Print and shaded views of the part. All mm, measured from the part's lowest x, y and z. Round coordinates to 2 decimals unless told otherwise and drop trailing zeros. Order: outer loops, then holes, each group sorted by start corner. A loop starts at its lowest first (then second) coordinate and runs counter-clockwise, first axis right, second up. Notation, with made-up numbers: (29.25, -3.5) - (39.25, -3.5) arc R17 cw to (39.25, 0.5) - close; hole circle Ø11 at (-37, 84.25). An arc over 180 degrees is marked (long way). Write item = value, one per line.
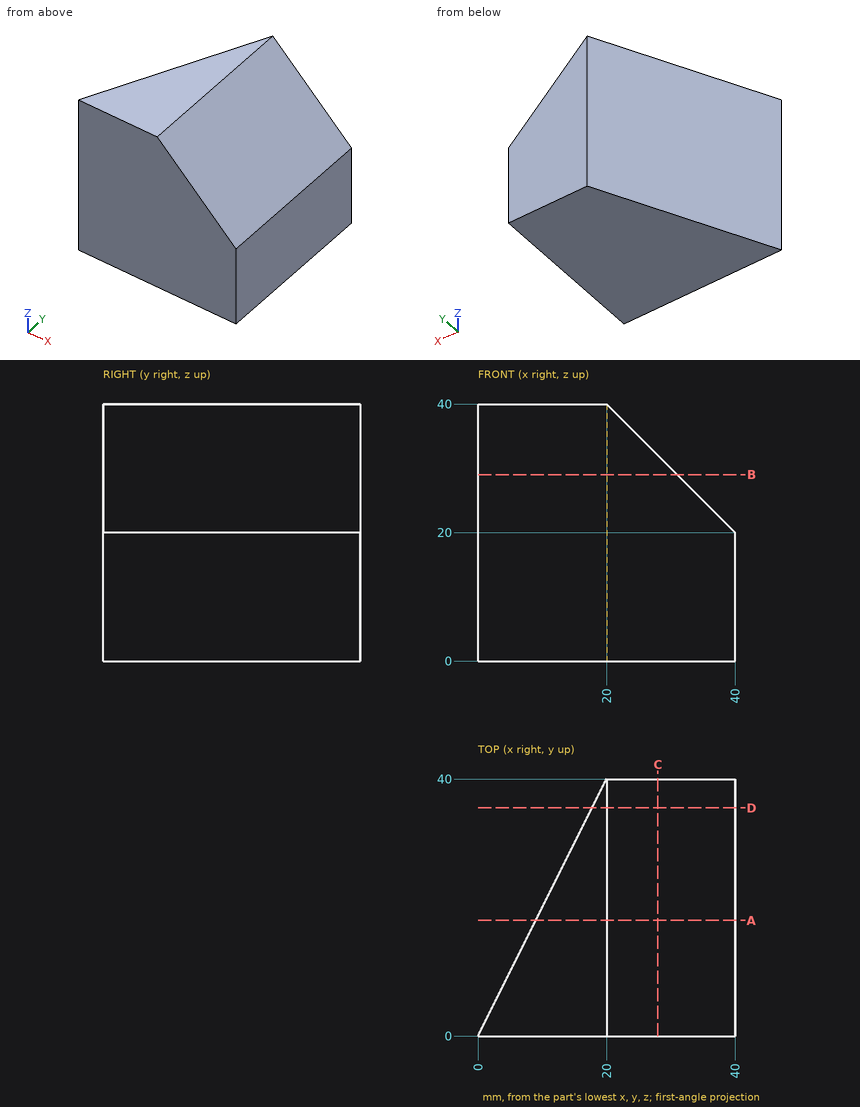
(1) Drop flat-ended pins along their axis: pin 1 (5 mm diameter, centred on y = 31.5, z = 5, fed in from -X); pin 2 (3 mm diameter, centred on y = 12.5, z = 21.5, fed in from -X). Give the stop position or say it passes through.
Solved:
pin_1 = 14.5
pin_2 = 5.5
(2) Band-saw the part on A-A on y = 18. List the corners of the cut face in (x, z).
Solved:
outline = (9, 0) - (40, 0) - (40, 20) - (20, 40) - (9, 40) - close
(3) Band-saw the part on B-B on z = 29. List the corners of the cut face in (x, y).
Solved:
outline = (0, 0) - (31, 0) - (31, 40) - (20, 40) - close
(4) Probe line 1 along X through (y, z) = (21.5, 2); line 2 along Y through (x, z) = (12.5, 20); line 3 along Z through (x, y) = (37, 23). List the from-to ranges inside material, lowest first.
Solved:
line_1 = 10.75 to 40
line_2 = 0 to 25
line_3 = 0 to 23
(5) Band-saw the part on C-C on x = 28. List the corners of the cut face in (y, z).
Solved:
outline = (0, 0) - (40, 0) - (40, 32) - (0, 32) - close
(6) Band-saw the part on D-D on y = 35.5. List the corners of the cut face in (x, z), plus the area to 3 significant figures.
Solved:
outline = (17.75, 0) - (40, 0) - (40, 20) - (20, 40) - (17.75, 40) - close
area = 690 mm²
